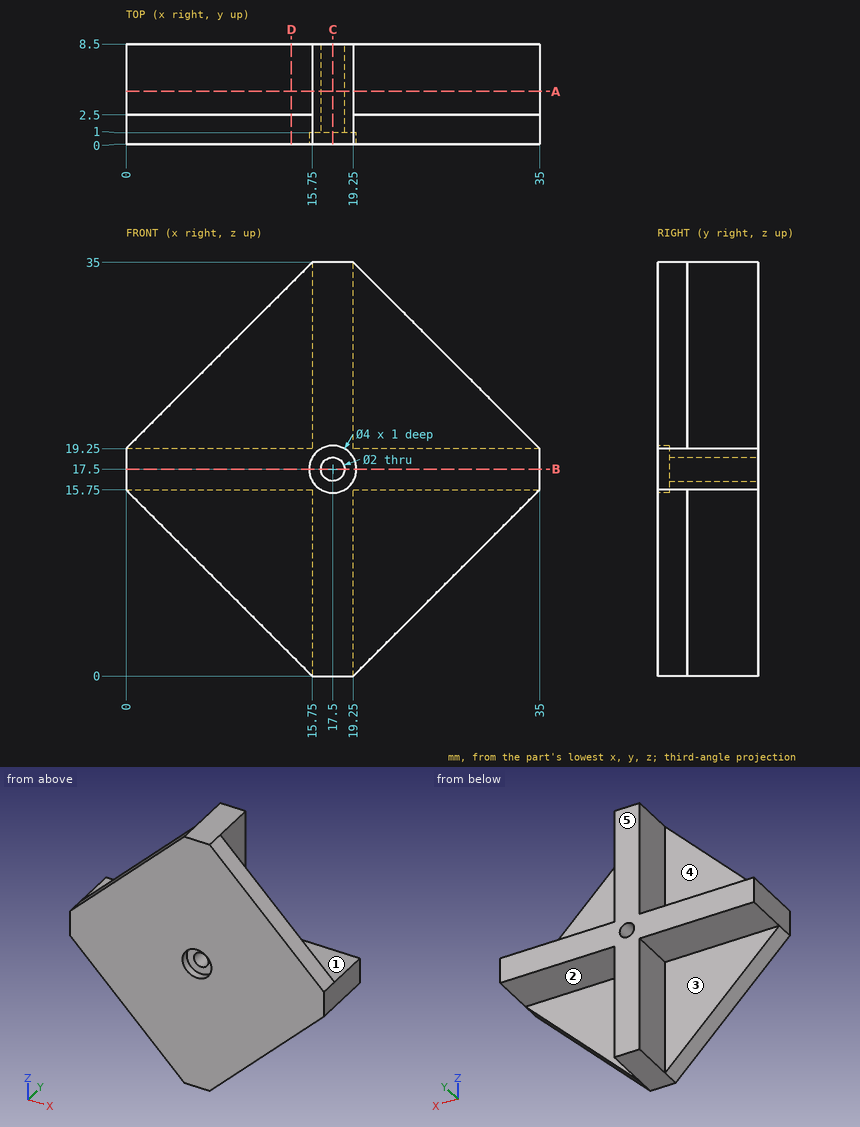
Answer from the drawing. Dimensions are ordinates in mm from the lowest x, y and z of the part. A direction names the side the tool comes from. Give positions to 0.01 mm unless a question says otherwise; leave off trailing zeros. Order: outer loops, then holes, each group sorted by start corner. A loop starts at its lowest first (then second) coordinate and runs counter-clockwise, first axis right, second up. Notation, with made-up numbers: (-32, 19.25) - (16, 19.25) arc R18 cw to (16, 30.25) - close; hole circle Ø9 at (-40, 68). An arc over 180 degrees is marked (long way). One line per item, written item: value. Start each with the question number.
1) A cutting plane is placed at D-D on x = 14. Give the vertices of the cut face in (y, z), then the cut area to 4 significant figures.
2) Given pin 1 Ø2 at (x, z) = (19.5, 8.5) entering from +Y; pin 2 Ø8 at (x, z) = (9, 7.5) entering from +Y; pin 3 Ø3 at (x, y) = (30.5, 4.5) entering from +Z; pin 4 Ø1.8 at (y, z) = (5.5, 10) entering from +X, each flat-ended and moving along its own axis, determine where each tip first touches the part or whether it passes through.
3) A tool of negligible diameter and unlimited length cuts with its end or side. For the marked faces 1, 2, 3, 4 and 5, from which of +Z, -Z, +X, -X, +Y, -Y can it reach the whole face along a straight path? Write none if from no direction.
4) A cutting plane is placed at A-A on y = 4.5. Give the vertices of the cut face in (x, z).
5) Find the intervals of material crossed by L1, parallel to Z at x = 17.5, y = 4.75; L2, parallel to Z at x = 3, y = 7, in increasing order.
6) A cutting plane is placed at C-C on x = 17.5. Give the vertices of the cut face in (y, z).
7) A cutting plane is placed at B-B on z = 17.5. Give the vertices of the cut face in (x, y), then the cut area to 4 significant figures.
Answer sheet:
1. outline: (0, 1.75) - (2.5, 1.75) - (2.5, 15.75) - (8.5, 15.75) - (8.5, 19.25) - (2.5, 19.25) - (2.5, 33.25) - (0, 33.25) - close
1. area: 99.75 mm2
2. pin 1: stops at y = 8.5
2. pin 2: stops at y = 2.5
2. pin 3: stops at z = 19.25
2. pin 4: stops at x = 19.25
3. face 1: +Z, +X, +Y
3. face 2: -Z, +X, +Y
3. face 3: -Z, -X, +Y
3. face 4: +Z, -X, +Y
3. face 5: +Z, -Z, +X, -X, +Y
4. outline: (0, 15.75) - (15.75, 15.75) - (15.75, 0) - (19.25, 0) - (19.25, 15.75) - (35, 15.75) - (35, 19.25) - (19.25, 19.25) - (19.25, 35) - (15.75, 35) - (15.75, 19.25) - (0, 19.25) - close; hole circle Ø2 at (17.5, 17.5)
5. L1: z = 0 to 16.5, 18.5 to 35
5. L2: z = 15.75 to 19.25
6. outline: (0, 0) - (8.5, 0) - (8.5, 16.5) - (1, 16.5) - (1, 15.5) - (0, 15.5) - close; (0, 19.5) - (1, 19.5) - (1, 18.5) - (8.5, 18.5) - (8.5, 35) - (0, 35) - close
7. outline: (0, 0) - (15.5, 0) - (15.5, 1) - (16.5, 1) - (16.5, 8.5) - (0, 8.5) - close; (18.5, 1) - (19.5, 1) - (19.5, 0) - (35, 0) - (35, 8.5) - (18.5, 8.5) - close
7. area: 278.5 mm2
